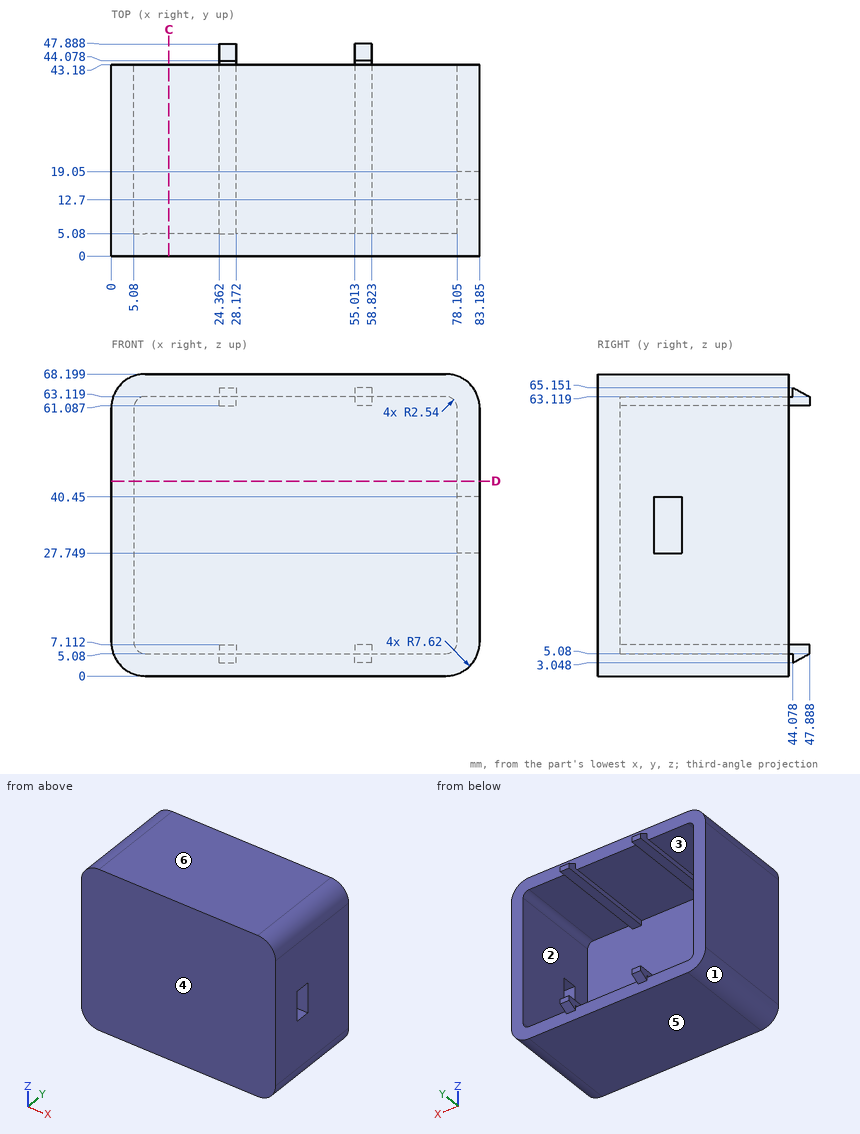
Print and shaded views of the part. All mm, measured from the part's lowest x, y and z. A direction names the side the tool comes from. Give positions to 0.01 mm unless a question says otherwise; leave off trailing zeros. Order: outer loops, then holes, each group sorted by start corner. A loop starts at its lowest first (then second) coordinate and runs counter-clockwise, first axis right, second up. Notation, with made-up numbers: (-35.75, 89) - (-17.75, 89) arc R15 ccw to (-17.75, 100) - close; hole circle Ø4 at (73.25, 32). An arc over 180 degrees is marked (long way). Use a Markdown table: item, result.
1) Saw through at D-D on z = 44. List the corners of the cut face in (x, y) (1 decimal).
Checked values:
| item | result |
|---|---|
| outline | (0, 0) - (83.2, 0) - (83.2, 43.2) - (78.1, 43.2) - (78.1, 5.1) - (5.1, 5.1) - (5.1, 43.2) - (0, 43.2) - close |
2) Two-plate mould, pull along Z, no slides. Class the marked faces 3, 4, 5 and 6: +Z half, -Z half, draft (parallel to the pull), parting line (faces both ways), or undercut.
Checked values:
| item | result |
|---|---|
| face 3 | undercut |
| face 4 | draft |
| face 5 | -Z half |
| face 6 | +Z half |
3) Saw through at C-C on x = 13. List the corners of the cut face in (y, z).
Checked values:
| item | result |
|---|---|
| outline | (0, 0) - (43.18, 0) - (43.18, 5.08) - (5.08, 5.08) - (5.08, 63.12) - (43.18, 63.12) - (43.18, 68.2) - (0, 68.2) - close |
4) Flat gauge pins, fed straight in: P1, Ø2, axis at y = 21.5, z = 5, coming from the -X side (1 decimal); P2, Ø4.5, axis at y = 17.5, z = 64, coming from the -X side; P3, Ø1.2, axis at y = 33.5, z = 63, coming from the +X side (1 decimal). Where does each tip first touch, or does it go through?
Checked values:
| item | result |
|---|---|
| P1 | x = 0.2 |
| P2 | x = 0.09 |
| P3 | x = 83 |
5) Probe L1, parallel to X at y = 42, z = 24 (1 decimal); L2, parallel to Z at x = 21.5, y = 39.5; L3, parallel to Z at x = 26.5, y = 19. List the from-to ranges inside material, lowest first. Write a range as from..to.
Checked values:
| item | result |
|---|---|
| L1 | 0..5.1, 78.1..83.2 |
| L2 | 0..5.08, 63.12..68.2 |
| L3 | 0..7.11, 61.09..68.2 |
6) 3-axis set-ups, long thin cutter, end or side, ignore diameter. For the marked faces 1 and 2: which of +Z, -Z, +X, -X, +Y, -Y reach the whole face in a straight line?
Checked values:
| item | result |
|---|---|
| face 1 | -Z, -X, +Y, -Y |
| face 2 | +Y |
